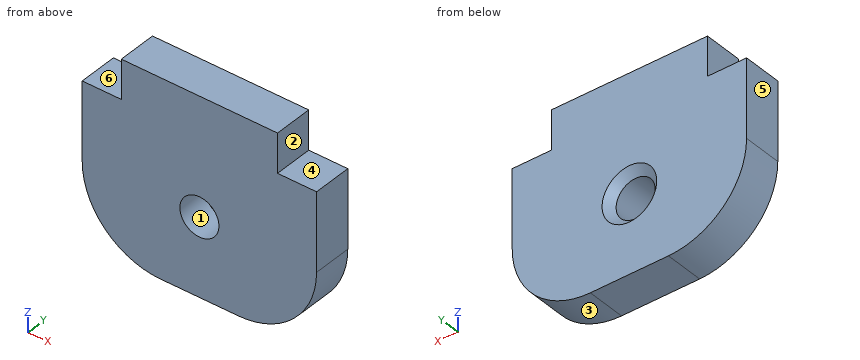
from build123d import *

# Parameters (mm, degrees)
EXTRUDE_1_DEPTH             = 5
HOLE_WIZARD_M61_D           = 5
HOLE_WIZARD_M61_CSINK_D     = 7
HOLE_WIZARD_M61_CSINK_ANGLE = 90


with BuildPart() as part:
    # Эскиз1 → Бобышка-Вытянуть1 (new body)
    with BuildSketch(Plane(origin=(0, 0, 0), x_dir=(1, 0, 0), z_dir=(0, 1, 0))):
        with BuildLine():
            Line((-15, 2.5), (-10, 2.5))
            Line((-10, 2.5), (-10, -2.5))
            Line((-10, -2.5), (10, -2.5))
            Line((10, -2.5), (10, 2.5))
            Line((10, 2.5), (15, 2.5))
            Line((15, 2.5), (15, 12.5))
            ThreePointArc((15, 12.5), (12.071067812, 19.571067812), (5, 22.5))
            Line((5, 22.5), (-5, 22.5))
            ThreePointArc((-5, 22.5), (-12.071067812, 19.571067812), (-15, 12.5))
            Line((-15, 12.5), (-15, 2.5))
        make_face()
    extrude(amount=EXTRUDE_1_DEPTH)

    # Отверстие обработанное метчиком M61 (through all)
    with Locations(Plane(origin=(0, 5, 0), x_dir=(1, 0, 0), z_dir=(0, 1, 0))):
        with Locations((0, 12.5)):
            CounterSinkHole(HOLE_WIZARD_M61_D / 2, HOLE_WIZARD_M61_CSINK_D / 2, counter_sink_angle=HOLE_WIZARD_M61_CSINK_ANGLE)


solid = part.part
Source: CAD feature listing. Evaluate the final solid. Frame: model axes, mm. Face numbers are marked on the shaded views. A direction names the side the tool comes from. Give positions to 0.01 mm unless a question says otherwise; leave off trailing zeros. Write each loop counter-clockwise with the first axis right and the second up, starting at its lowest first coordinate (ties: lowest second). Pieces come first, ordered by that corner, then holes. Notation, with made-up numbers: (59, 27.25) -> (103, 27.25) arc R17 cw to (103, 52.25) -> close; hole circle Ø2 at (4, 12.25). An arc over 180 degrees is marked (long way). Return JSON: item names as keys, results as strings. Group by question number.
1. Section A-A, the plane x = 0. Output: boundary loops of the cut face in (y, z), then the cut area to 3 significant figures.
2. Material intervals for line 1 (X direction, y = 1.2, z = -12.5); line 2 (Z direction, x = 0, y = 1.4); line 3 (Z direction, x = -1, y = 2.75), sorted ascending. Write a range as from..to.
3. Pin query (flat end, axial travel): pin 1 Ø2.5 at (x, y) = (-13, 3) entering from +Z; pin 2 Ø1 at (x, z) = (-6, -1.5) entering from -Y; pin 3 Ø2.5 at (y, z) = (3, 0.5) entering from -X. Return the tip coordinate at first contact, or that it passes through.
4. Section B-B, the plane y = 1.3. Output: boundary loops of the cut face in (x, z), then the cut area to 3 significant figures.
5. Access query for the marked faces 4, 5 and 6. Directions: +Z, -Z, +X, -X, +Y, -Y. A direction counts if a zero-diameter tool reaches every point of the face in a straight line with its end or side. Return the directions, or none.
6. Mould query, pull axis Z, two halves, no side actions, for the marked faces 1, 2 and 3. Classes: +Z half, -Z half, draft (parallel to the pull), parting line (faces both ways), or undercut.
Determined:
{
 "1": {"outline": "(0, -22.5) -> (5, -22.5) -> (5, -16) -> (4, -15) -> (0, -15) -> close; (0, -10) -> (4, -10) -> (5, -9) -> (5, 2.5) -> (0, 2.5) -> close", "area": "99.0 mm2"},
 "2": {"line 1": "x = -15..-2.5, 2.5..15", "line 2": "z = -22.5..-15, -10..2.5", "line 3": "z = -22.5..-14.79, -10.21..2.5"},
 "3": {"pin 1": "stops at z = -2.5", "pin 2": "stops at y = 0", "pin 3": "stops at x = -10"},
 "4": {"outline": "(-15, -12.5) arc R10 ccw to (-5, -22.5) -> (5, -22.5) arc R10 ccw to (15, -12.5) -> (15, -2.5) -> (10, -2.5) -> (10, 2.5) -> (-10, 2.5) -> (-10, -2.5) -> (-15, -2.5) -> close; hole circle Ø5 at (0, -12.5)", "area": "637 mm2"},
 "5": {"face 4": "+Z, +X, +Y, -Y", "face 5": "+Z, -Z, -X, +Y, -Y", "face 6": "+Z, -X, +Y, -Y"},
 "6": {"face 1": "undercut", "face 2": "draft", "face 3": "-Z half"}
}
